Could you check a few things on this model? Use its own coordinates, in mm. Face numbers are marked on the shaded views. A direction names the side the tool comes from. Coordinates: 2 decimals unless noted, no trailing zeros. Loops run counter-clockwise (first coordinate to the right, second up) from the corner with the lowest first, then second, coordinate; pieces in that order, holes last.
1) Imagine slicing it at C-C on x = -110. Please give me the cut outline in (y, z), plus the area to 3 significant figures.
2) Imagine slicing it at D-D on y = -41.5. Please give me the cut outline in (x, z).
3) Imagine slicing it at B-B on x = -33.5. Please give me the cut outline in (y, z), plus the area to 3 significant figures.
4) Imagine slicing it at A-A on y = -22. Please give me the cut outline in (x, z).
5) For the marked faces 1, 2, 3, 4 and 5, which set-ups out of +Z, -Z, +X, -X, +Y, -Y let a thin tool reach every point of the face, with its end or its side?
6) Will these pins go through, and if not, where does the flat tip stop? P1, Ø10, axis at y = -7.5, z = -8.5, coming from the -X side; P2, Ø20, axis at x = -49, z = 0, coming from the -Y side; P3, Ø6.5, axis at x = -33.5, z = -15.5, coming from the -Y side; P4, Ø9.5, axis at x = -110, y = -13.5, coming from the -Z side.
7) If I drill on line 1 along Z through (x, y) = (-64.5, -1.15); line 2 along Z through (x, y) = (-110, -1); line 3 along X through (y, z) = (-0.65, 0), over which ranges is the centre line in solid material (lowest first)?
8) Thinking about a two-plate mould opening in X: for the marked faces 6, 7 and 8, which applies, released by +X, released by -X, zero draft, split by the parting line, or undercut?
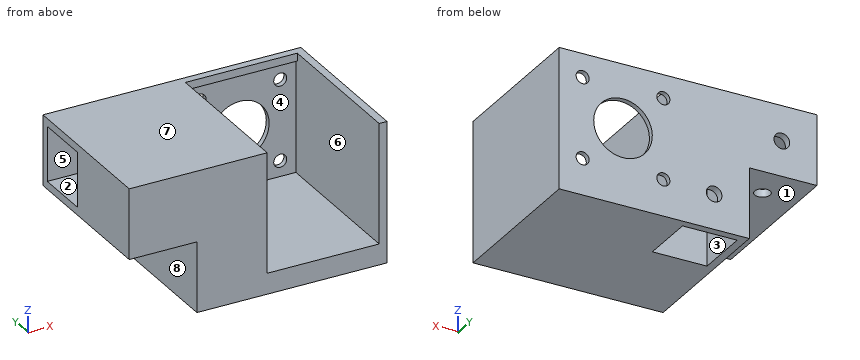
```python
from build123d import *

# Parameters (mm, degrees)
SKETCH1_R           = 2.5
SKETCH1_R_2         = 11.25
BOSS_EXTRUDE1_DEPTH = 60
SKETCH2_W           = 43
SKETCH2_H           = 43
CUT_EXTRUDE1_DEPTH  = 58
SKETCH3_W           = 21
SKETCH3_H           = 21
CUT_EXTRUDE2_DEPTH  = 51
SKETCH4_W           = 21
SKETCH4_H           = 21
CUT_EXTRUDE3_DEPTH  = 50
CUT_EXTRUDE5_REACH  = 100.991
SKETCH6_R           = 3
CUT_EXTRUDE6_REACH  = 102.102
SKETCH7_R           = 3
CUT_EXTRUDE7_REACH  = 101.394
SKETCH8_R           = 3
CUT_EXTRUDE8_REACH  = 102.102
SKETCH9_R           = 3
CUT_EXTRUDE9_REACH  = 149.541
SKETCH10_W          = 43
SKETCH10_H          = 57


with BuildPart() as part:
    # Sketch1 → Boss-Extrude1 (new body)
    with BuildSketch(Plane(origin=(0, 0, 0), x_dir=(1, 0, 0), z_dir=(0, 1, 0))):
        Polygon((-24.5, 29.5), (48.5, 29.5), (48.5, 2.5), (74.5, 2.5), (74.5, -24.5), (48.5, -24.5), (-24.5, -24.5), align=None)
        with Locations(Location((15.5, 15.5, 0), (0, 0, 270))):
            Circle(SKETCH1_R, mode=Mode.SUBTRACT)
        with Locations(Location((-15.5, 15.5, 0), (0, 0, 270))):
            Circle(SKETCH1_R, mode=Mode.SUBTRACT)
        with Locations(Location((15.5, -15.5, 0), (0, 0, 270))):
            Circle(SKETCH1_R, mode=Mode.SUBTRACT)
        with Locations(Location((-15.5, -15.5, 0), (0, 0, 270))):
            Circle(SKETCH1_R, mode=Mode.SUBTRACT)
        with Locations(Location((0, 0, 0), (0, 0, 270))):
            Circle(SKETCH1_R_2, mode=Mode.SUBTRACT)
    extrude(amount=-BOSS_EXTRUDE1_DEPTH)

    # Sketch2 → Cut-Extrude1 (cut)
    with BuildSketch(Plane.XZ.offset(60)):
        Rectangle(SKETCH2_W, SKETCH2_H)
    extrude(amount=-CUT_EXTRUDE1_DEPTH, mode=Mode.SUBTRACT)

    # Sketch3 → Cut-Extrude2 (cut)
    with BuildSketch(Plane(origin=(0, 0, -29.5), x_dir=(-1, 0, 0), z_dir=(0, 0, -1))):
        with Locations((-35, -13.5)):
            Rectangle(SKETCH3_W, SKETCH3_H)
    extrude(amount=-CUT_EXTRUDE2_DEPTH, mode=Mode.SUBTRACT)

    # Sketch4 → Cut-Extrude3 (cut)
    with BuildSketch(Plane(origin=(74.5, 0, 0), x_dir=(0, 0, -1), z_dir=(1, 0, 0))):
        with Locations((-11, -13.5)):
            Rectangle(SKETCH4_W, SKETCH4_H)
    extrude(amount=-CUT_EXTRUDE3_DEPTH, mode=Mode.SUBTRACT)

    # Sketch6 → Cut-Extrude5 (cut, up to next)
    with BuildSketch(Plane(origin=(48.5, 0, 0), x_dir=(0, 0, -1), z_dir=(1, 0, 0)), mode=Mode.PRIVATE) as cut_extrude5_sk1:
        with Locations((16, -13.5)):
            Circle(SKETCH6_R)
    cut_extrude5_tool1 = extrude(cut_extrude5_sk1.sketch, amount=-CUT_EXTRUDE5_REACH, mode=Mode.PRIVATE) & part.part
    add(cut_extrude5_tool1.solids().sort_by_distance((48.5, -13.5, -16))[0], mode=Mode.SUBTRACT)

    # Sketch7 → Cut-Extrude6 (cut, up to next)
    with BuildSketch(Plane(origin=(0, 0, 0), x_dir=(1, 0, 0), z_dir=(0, 1, 0)), mode=Mode.PRIVATE) as cut_extrude6_sk1:
        with Locations(Location((35, 16, 0), (0, 0, 270))):
            Circle(SKETCH7_R)
    cut_extrude6_tool1 = extrude(cut_extrude6_sk1.sketch, amount=-CUT_EXTRUDE6_REACH, mode=Mode.PRIVATE) & part.part
    add(cut_extrude6_tool1.solids().sort_by_distance((35, 0, -16))[0], mode=Mode.SUBTRACT)

    # Sketch8 → Cut-Extrude7 (cut, up to next)
    with BuildSketch(Plane(origin=(0, 0, -2.5), x_dir=(-1, 0, 0), z_dir=(0, 0, -1)), mode=Mode.PRIVATE) as cut_extrude7_sk1:
        with Locations((-61, -13.5)):
            Circle(SKETCH8_R)
    cut_extrude7_tool1 = extrude(cut_extrude7_sk1.sketch, amount=-CUT_EXTRUDE7_REACH, mode=Mode.PRIVATE) & part.part
    add(cut_extrude7_tool1.solids().sort_by_distance((61, -13.5, -2.5))[0], mode=Mode.SUBTRACT)

    # Sketch9 → Cut-Extrude8 (cut, up to next)
    with BuildSketch(Plane(origin=(0, 0, 0), x_dir=(1, 0, 0), z_dir=(0, 1, 0)), mode=Mode.PRIVATE) as cut_extrude8_sk1:
        with Locations(Location((61, -11, 0), (0, 0, 270))):
            Circle(SKETCH9_R)
    cut_extrude8_tool1 = extrude(cut_extrude8_sk1.sketch, amount=-CUT_EXTRUDE8_REACH, mode=Mode.PRIVATE) & part.part
    add(cut_extrude8_tool1.solids().sort_by_distance((61, 0, 11))[0], mode=Mode.SUBTRACT)


with BuildPart() as body_2:
    # Mirror3: mirrored copy
    add(part.part.mirror(Plane(origin=(-24.5, -60, 0), x_dir=(0, 0, 1), z_dir=(-1, 0, 0))))

    # Sketch10 → Cut-Extrude9 (cut, up to next)
    with BuildSketch(Plane.XY.offset(24.5), mode=Mode.PRIVATE) as cut_extrude9_sk1:
        with Locations((-49, -31.5)):
            Rectangle(SKETCH10_W, SKETCH10_H)
    cut_extrude9_tool1 = extrude(cut_extrude9_sk1.sketch, amount=-CUT_EXTRUDE9_REACH, mode=Mode.PRIVATE) & body_2.part
    add(cut_extrude9_tool1.solids().sort_by_distance((-49, -31.5, 24.5))[0], mode=Mode.SUBTRACT)


solid = body_2.part
```
Filled in:
1. outline: (-60, -2.5) - (-16.5, -2.5) - (-16.5, 0.5) - (-24, 0.5) - (-24, 21.5) - (-3, 21.5) - (-3, 14) - (0, 14) - (0, 24.5) - (-60, 24.5) - close; (-10.5, -2.5) - (0, -2.5) - (0, 8) - (-3, 8) - (-3, 0.5) - (-10.5, 0.5) - close
1. area: 1,140 mm2
2. outline: (-123.5, -2.5) - (-97.5, -2.5) - (-97.5, -29.5) - (-24.5, -29.5) - (-24.5, 24.5) - (-27.5, 24.5) - (-27.5, -21.5) - (-70.5, -21.5) - (-70.5, 24.5) - (-123.5, 24.5) - close
3. outline: (-60, -29.5) - (0, -29.5) - (0, -18) - (-2, -18) - (-2, -21.5) - (-60, -21.5) - close; (-3, 21.5) - (-2, 21.5) - (-2, 18) - (0, 18) - (0, 24.5) - (-3, 24.5) - close; (-2, -13) - (0, -13) - (0, 13) - (-2, 13) - close
3. area: 555 mm2
4. outline: (-123.5, -2.5) - (-97.5, -2.5) - (-97.5, -29.5) - (-94.5, -29.5) - (-94.5, 0.5) - (-123.5, 0.5) - close; (-123.5, 21.5) - (-73.5, 21.5) - (-73.5, -29.5) - (-24.5, -29.5) - (-24.5, 24.5) - (-27.5, 24.5) - (-27.5, -21.5) - (-70.5, -21.5) - (-70.5, 24.5) - (-123.5, 24.5) - close
5. face 1: -Z, -X, +Y, -Y
5. face 2: -X
5. face 3: -Z
5. face 4: -Y
5. face 5: none
6. P1: stops at x = -97.5
6. P2: passes through
6. P3: stops at y = -2
6. P4: stops at z = -2.5
7. line 1: z = -29.5 to -18, -13 to 13, 18 to 24.5
7. line 2: z = -2.5 to 8, 14 to 24.5
7. line 3: x = -123.5 to -60.25, -37.75 to -24.5
8. face 6: undercut
8. face 7: zero draft
8. face 8: released by -X
